Read the model definition and answer for the solid it produces. Units are mm, in the model's axes. Face numbers are marked on the shaded views. A direction names the side the tool comes from. Round coordinates to 2 decimals unless told otherwise and drop trailing zeros. Loops run counter-clockwise (first coordinate to the right, second up) from the corner with the lowest first, then second, coordinate; pieces in that order, holes last. Notation, with made-up numbers: M -13.75,48 L 33.25,48 A22 ccw 33.25,54 Z; hole C 19,-23.75 d5. An arc over 180 degrees is marked long. Answer as CSV lines item,"result".
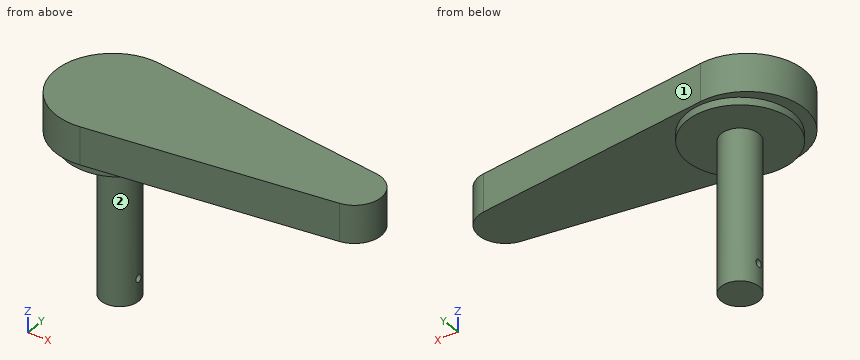
Solid Edge part; units mm, degrees
sketch "Sketch1" plane through (0, 0, 0) normal (0, 0, 1) x (1, 0, 0)
  line L0 (63, 7) -> (0, 15)
  arc A0 (0, 15) -> (0, -15) centre (-1.9048, 0) ccw
  line L1 (63, -7) -> (0, -15)
  arc A1 (63, 7) -> (63, -7) centre (62.1111, 0) cw
extrude "Protrusion1" add sketch "Sketch1" along normal blind 10
sketch "Sketch2" plane through (26.0711, 0, 0) normal (0, 0, -1) x (-0.992, -0.126, 0)
  circle A0 centre (25.8634, 3.2842) radius 5
extrude "ExtrudedProtrusion_2" add sketch "Sketch2" along normal blind 42
sketch "Sketch3" plane through (0, 0, 0) normal (1, 0, 0) x (0, 1, 0)
  circle A0 centre (0, -36) radius 1
extrude "Cutout1" cut sketch "Sketch3" along normal mid plane 36.7222
sketch "Sketch4" plane through (26.0711, 0, 0) normal (0, 0, -1) x (-0.992, -0.126, 0)
  circle A0 centre (25.8634, 3.2842) radius 14
extrude "ExtrudedProtrusion_3" add sketch "Sketch4" along normal blind 2
1) Find section D-D, the plane z = -28. Give the vertices of the cut face in (x, y).
Evaluation:
outline,"C 0,0 d10"
2) Each of these flat-tipped pins is pushed along its axis until it touches: P1, Ø10, axis at x = 32.5, z = 4.5, coming from the -Y side; P2, Ø8.5, axis at x = 2.5, y = 7, coming from the -Z side; P3, Ø4, axis at y = 6.5, z = -32.5, coming from the +X side; P4, Ø10, axis at x = 20.5, y = 3.5, coming from the -Z side. Where does it stop, or does it pass through?
Evaluation:
P1,"stops at y = -11.51"
P2,"stops at z = -42"
P3,"stops at x = 2.18"
P4,"stops at z = 0"
3) A tool of negligible diameter and unlimited length cuts with its end or side. For the marked faces 1 and 2, from which of +Z, -Z, +X, -X, +Y, -Y can it reach the whole face along a straight path? Write none if from no direction.
Evaluation:
face 1,"+Z, -Z, +X, +Y"
face 2,"-Z"
4) Find section C-C, the plane x = 42. Give the vertices of the cut face in (y, z), then the cut area to 3 significant figures.
Evaluation:
outline,"M -9.67,0 L 9.67,0 L 9.67,10 L -9.67,10 Z"
area,"193 mm^2"
5) Find section B-B, the plane y = -13. Give the vertices of the cut face in (x, z), then the cut area to 3 significant figures.
Evaluation:
outline,"M -9.63,0 L -5.2,0 L -5.2,-2 L 5.2,-2 L 5.2,0 L 15.75,0 L 15.75,10 L -9.63,10 Z"
area,"275 mm^2"
6) Find section A-A, the plane z = 3. Give the vertices of the cut face in (x, y).
Evaluation:
outline,"M 0,-15 L 63,-7 A7.06 ccw 63,7 L 0,15 A15.12 ccw long Z"
7) Straight lines are drawn through the part: line 1 (Z direction, x = 1.75, y = 0); line 2 (Y direction, x = 1.25, z = -36); line 3 (Y direction, x = -1, z = -36). For each, find the intervals that lie inside material, in ascending order.
Evaluation:
line 1,"z = -42 to -37, -35 to 10"
line 2,"y = -4.84 to -1, 1 to 4.84"
line 3,"y = -4.9 to -1, 1 to 4.9"
